Input: part model. Units: mm. Frame: model coordinates. A direction names the side the tool comes from. Round coordinates to 2 decimals unless told otherwise and drop trailing zeros. Write each loop counter-clockwise with the first axis right and the second up, starting at its lowest first coordinate (ties: lowest second). Pieces come first, ordered by that corner, then holes. Notation, with made-up numbers: (3.5, 32) - (17.5, 32) arc R22 cw to (17.5, 49) - close; hole circle Ø8 at (2.25, 2.5). An arc over 180 degrees is marked (long way). Use one line per item in the form item = value.
```python
from build123d import *

# Parameters (mm, degrees)
F0_R         = 9.525
F0_R_2       = 1.5875
F1_DEPTH     = 2.54
F2_R         = 9.525
F2_R_2       = 7.62
F3_DEPTH     = 3.175
F4_R         = 9.525
F4_R_2       = 7.747
F5_DEPTH     = 2.54
F6_R         = 3.175
F7_DEPTH     = 12.7
F10_R        = 2.54
F11_DEPTH    = 27.9544081902
F12_T2_ANGLE = 180
F12_T4_ANGLE = 180


# Not quite as in the source:
# - a fillet or chamfer that OpenCascade refuses, or shapes differently, is made with other operations: its cross-section is extruded or revolved along the edge and cut away or added


with BuildPart() as f1:
    # F0 (on Front) → F1 (new body)
    with BuildSketch(Plane.XZ):
        Circle(F0_R)
        with Locations((-4.3994090512, -2.54)):
            Circle(F0_R_2, mode=Mode.SUBTRACT)
        with Locations((4.3994090512, -2.54)):
            Circle(F0_R_2, mode=Mode.SUBTRACT)
        with Locations((0, 5.08)):
            Circle(F0_R_2, mode=Mode.SUBTRACT)
    extrude(amount=F1_DEPTH)

    # F2 (on face) → F3 (join)
    with BuildSketch(Plane.XZ.offset(2.54)):
        Circle(F2_R)
        Circle(F2_R_2, mode=Mode.SUBTRACT)
    extrude(amount=F3_DEPTH)

    # F4 (on face) → F5 (join)
    with BuildSketch(Plane(origin=(0, 0, 0), x_dir=(-1, 0, 0), z_dir=(0, 1, 0))):
        Circle(F4_R)
        Circle(F4_R_2, mode=Mode.SUBTRACT)
    extrude(amount=F5_DEPTH)

    # F6 (on face) → F7 (join)
    with BuildSketch(Plane(origin=(0, 0, 0), x_dir=(-1, 0, 0), z_dir=(0, 1, 0))):
        Circle(F6_R)
    extrude(amount=F7_DEPTH)

    # F8 (on Top) → F9 (revolve)
    with BuildSketch(Plane.XY):
        with BuildLine():
            Line((0, 27.9505403934), (0, 9.2075))
            ThreePointArc((0, 9.2075), (9.6048581812, 16.9002312755), (4.1957274517, 27.9534081902))
            Line((4.1957274517, 27.9534081902), (0, 27.9505403934))
        make_face()
    revolve(axis=Axis((0, 12.9395495169, 0), (0, -1, 0)))

    # F10 (on face) → F11 (cut, through all)
    with BuildSketch(Plane(origin=(0, 0, 0), x_dir=(-1, 0, 0), z_dir=(0, 1, 0))):
        Circle(F10_R)
    extrude(amount=F11_DEPTH, mode=Mode.SUBTRACT)

    # F12: chamfer of 3.81 on 2 edges, made by hand

    # F12_s1 → F12_t2 (revolve)
    with BuildSketch(Plane.XY):
        with BuildLine():
            Line((-3.1035480311, 6.3541505323), (-5.586882311, 11.0326284828))
            Line((-5.586882311, 11.0326284828), (-5.5441822052, 11.0957406129))
            ThreePointArc((-5.5441822052, 11.0957406129), (-4.405806786, 10.3339526014), (-3.1504193548, 9.8057870222))
            Line((-3.1504193548, 9.8057870222), (-3.0988, 9.733660523))
            ThreePointArc((-3.0988, 9.733660523), (-3.0988, 8.0439055277), (-3.0273480311, 6.3541505323))
            Line((-3.0273480311, 6.3541505323), (-3.1035480311, 6.3541505323))
        make_face()
    revolve(axis=Axis((0, 9.733660523, 0), (0, -1, 0)), revolution_arc=F12_T2_ANGLE)

    # F12_s3 → F12_t4 (revolve)
    with BuildSketch(Plane.XY):
        with BuildLine():
            Line((3.1035480311, 6.3541505323), (5.586882311, 11.0326284828))
            Line((5.586882311, 11.0326284828), (5.5441822052, 11.0957406129))
            ThreePointArc((5.5441822052, 11.0957406129), (4.405806786, 10.3339526014), (3.1504193548, 9.8057870222))
            Line((3.1504193548, 9.8057870222), (3.0988, 9.733660523))
            ThreePointArc((3.0988, 9.733660523), (3.0988, 8.0439055277), (3.0273480311, 6.3541505323))
            Line((3.0273480311, 6.3541505323), (3.1035480311, 6.3541505323))
        make_face()
    revolve(axis=Axis((0, 9.733660523, 0), (0, -1, 0)), revolution_arc=F12_T4_ANGLE)


solid = f1.part
```
(1) Access query for faces 1 (the face through (0.69, 3.2, -3.1)), 2 (the face through (0, -2.54, 0)), 3 (the face through (0.33, 13.78, 2.52)). Directions: +Z, -Z, +X, -X, +Y, -Y. A direction counts if a zero-diameter tool reaches every point of the face in a straight line with its end or side. Return the directions, or none.
Derived:
face_1 = none
face_2 = -Y
face_3 = +Y
(2) Cut plane B-B on z = 6. Output: boundary loops of the cut face in (x, y) (3 decimals).
Derived:
outline = circle Ø15.604 at (0, 19.05); (-7.398, -5.715) - (-4.697, -5.715) - (-4.697, -2.54) - (-1.294, -2.54) - (-1.294, 0) - (-4.901, 0) - (-4.901, 2.54) - (-7.398, 2.54) - close; (1.294, -2.54) - (4.697, -2.54) - (4.697, -5.715) - (7.398, -5.715) - (7.398, 2.54) - (4.901, 2.54) - (4.901, 0) - (1.294, 0) - close
(3) Draft query along X for faces 4 (the face through (-0.72, 6.76, -3.24)), 5 (the face through (0, -5.715, 8)), 6 (the face through (3.33, 0, 0.11)). Return one class per face: released by +X, released by -X, zero draft, split by the parting line, or undercut.
Derived:
face_4 = split by the parting line
face_5 = zero draft
face_6 = undercut
(4) Cut plane C-C on y = -2. Count the separate pieces of the cut face and the enclosed holes in it, then the cut area to 3 significant figures.
Derived:
separate_pieces = 1
enclosed_holes = 3
area = 261 mm^2
(5) First-contact query: pin 1 Ø4 at (x, z) = (0, 0) entering from +Y; pin 2 Ø4.5 at (x, z) = (-0.5, 1) entering from -Y; pin 3 Ø1.5 at (x, y) = (0.5, 6) entering from +Z. Flat tips, straight axial feed; report the tip coordinate or a pass-through.
Derived:
pin_1 = 0
pin_2 = -2.54
pin_3 = 3.29
(6) Material intervals for L1, parallel to Z at x = 0, y = -4.7 (3 decimals); L2, parallel to Z at x = 0, y = 0.5 (3 decimals); L3, parallel to Z at x = 0, y = 6.25 (3 decimals), sorted ascending.
Derived:
L1 = -9.525 to -7.62, 7.62 to 9.525
L2 = -9.525 to -7.747, -3.175 to -2.54, 2.54 to 3.175, 7.747 to 9.525
L3 = -3.175 to -2.54, 2.54 to 3.175
